```python
from build123d import *

# Parameters (mm, degrees)
SKETCH1_W    = 12
SKETCH1_H    = 12
NUCLEO_DEPTH = 12
SKETCH2_W    = 42
SKETCH2_H    = 2.5
SKETCH3_W    = 29
SKETCH3_H    = 2.5


with BuildPart() as part:
    # Sketch1 → Nucleo (new body)
    with BuildSketch(Plane.XY.offset(-6)):
        Rectangle(SKETCH1_W, SKETCH1_H)
    extrude(amount=NUCLEO_DEPTH)

    # Sketch2 → Eje_flexion (revolve)
    with BuildSketch(Plane.XY, mode=Mode.PRIVATE) as eje_flexion_sk:
        with Locations((0, 1.25)):
            Rectangle(SKETCH2_W, SKETCH2_H)
    revolve(eje_flexion_sk.sketch.rotate(Axis((-25, 0, 0), (1, 0, 0)), 90), axis=Axis((-25, 0, 0), (1, 0, 0)))

    # Sketch3 → Eje_desviacion (revolve)
    with BuildSketch(Plane(origin=(0, 0, 0), x_dir=(0, 0, -1), z_dir=(1, 0, 0)), mode=Mode.PRIVATE) as eje_desviacion_sk:
        with Locations((0, 1.25)):
            Rectangle(SKETCH3_W, SKETCH3_H)
    revolve(eje_desviacion_sk.sketch.rotate(Axis((0, 0, 18.5), (0, 0, -1)), 90), axis=Axis((0, 0, 18.5), (0, 0, -1)))


solid = part.part
```
Geometry check sheet. Reference: the model listing, model coordinates, mm. A direction names the side the tool comes from. Coordinates: 2 decimals unless noted, no trailing zeros. Order: outer loops, then holes, each group sorted by start corner. A loop starts at its lowest first (then second) coordinate and runs counter-clockwise, first axis right, second up. Notation, with made-up numbers: (-28, -8) - (22, -8) arc R19 ccw to (22, 23) - close; hole circle Ø6 at (21, 40.25). An arc over 180 degrees is marked (long way). Answer in a Markdown table with one row per item. Add a question column.
1. Section check A-A (x = 0). Enter the section's corners in (y, z).
2. Section check C-C (z = -2). Enter the section's corners in (x, y), plus the area to 3 significant figures.
3. Material ranges on L1, parallel to X at y = -1.25, z = -2.75; L2, parallel to Y at x = 16, z = 2, recorded low to high. Write a range as [from, to].
4. Gauge pin test, flat ends, axial feed: pin 1 Ø4 at (x, y) = (13.5, 4) entering from +Z; pin 2 Ø4 at (x, y) = (7, 3.5) entering from +Z; pin 3 Ø4 at (x, y) = (14.5, -3.5) entering from -Z. Record the tip position at first contact, or that the pin passes through.
5. Access from +Z, -Z, +X, -X, +Y, -Y to the whole of each face (thin tool, end or side, straight path). Record for faces 1 (the face through (3, 0, -6)), 2 (the face through (-13.4, -0.1, -2.5)), 3 (the face through (3, 0, 6)).
6. Section check B-B (y = 2). Enter the section's corners in (x, z), plus the area to 3 significant figures.
7. Section check D-D (y = 0). Enter the section's corners in (x, z), plus the area to 3 significant figures.
Data:
| question | item | result |
|---|---|---|
| 1 | outline | (-6, -6) - (-2.5, -6) - (-2.5, -14.5) - (2.5, -14.5) - (2.5, -6) - (6, -6) - (6, 6) - (2.5, 6) - (2.5, 14.5) - (-2.5, 14.5) - (-2.5, 6) - (-6, 6) - close |
| 2 | outline | (-21, -1.5) - (-6, -1.5) - (-6, -6) - (6, -6) - (6, -1.5) - (21, -1.5) - (21, 1.5) - (6, 1.5) - (6, 6) - (-6, 6) - (-6, 1.5) - (-21, 1.5) - close |
| 2 | area | 234 mm² |
| 3 | L1 | x = [-6, 6] |
| 3 | L2 | y = [-1.5, 1.5] |
| 4 | pin 1 | stops at z = 1.5 |
| 4 | pin 2 | stops at z = 6 |
| 4 | pin 3 | stops at z = -2 |
| 5 | face 1 | -Z |
| 5 | face 2 | -X |
| 5 | face 3 | +Z |
| 6 | outline | (-21, -1.5) - (-6, -1.5) - (-6, -6) - (-1.5, -6) - (-1.5, -14.5) - (1.5, -14.5) - (1.5, -6) - (6, -6) - (6, -1.5) - (21, -1.5) - (21, 1.5) - (6, 1.5) - (6, 6) - (1.5, 6) - (1.5, 14.5) - (-1.5, 14.5) - (-1.5, 6) - (-6, 6) - (-6, 1.5) - (-21, 1.5) - close |
| 6 | area | 285 mm² |
| 7 | outline | (-21, -2.5) - (-6, -2.5) - (-6, -6) - (-2.5, -6) - (-2.5, -14.5) - (2.5, -14.5) - (2.5, -6) - (6, -6) - (6, -2.5) - (21, -2.5) - (21, 2.5) - (6, 2.5) - (6, 6) - (2.5, 6) - (2.5, 14.5) - (-2.5, 14.5) - (-2.5, 6) - (-6, 6) - (-6, 2.5) - (-21, 2.5) - close |
| 7 | area | 379 mm² |
